```python
from build123d import *

# Parameters (mm, degrees)
ESQUISSE1_W        = 45
ESQUISSE1_H        = 60
BOSS_EXTRU_1_DEPTH = 5


with BuildPart() as part:
    # Esquisse1 → Boss.-Extru.1 (new body)
    with BuildSketch(Plane.XY):
        Polygon((112.625631329, 137.374368671), (100, 150), (-100, 150), (-112.625631329, 137.374368671), (-98.483495706, 123.232233047), (-123.232233047, 98.483495706), (-137.374368671, 112.625631329), (-150, 100), (-150, -100), (-137.374368671, -112.625631329), (-123.232233047, -98.483495706), (-98.483495706, -123.232233047), (-112.625631329, -137.374368671), (-100, -150), (100, -150), (112.625631329, -137.374368671), (98.483495706, -123.232233047), (123.232233047, -98.483495706), (137.374368671, -112.625631329), (150, -100), (150, 100), (137.374368671, 112.625631329), (123.232233047, 98.483495706), (98.483495706, 123.232233047), align=None)
        Rectangle(ESQUISSE1_W, ESQUISSE1_H, mode=Mode.SUBTRACT)
    extrude(amount=BOSS_EXTRU_1_DEPTH)


solid = part.part
```
Work out the finished part from the listing and answer in its coordinate system (mm). A direction names the side the tool comes from. Round coordinates to 2 decimals unless told otherwise and drop trailing zeros. Order: outer loops, then holes, each group sorted by start corner. A loop starts at its lowest first (then second) coordinate and runs counter-clockwise, first axis right, second up.
Q1. A cutting plane is placed at C-C, the plane z = 2.5. Determine the outline of the cut face in (x, y).
Solution:
outline: (-150, -100) - (-137.37, -112.63) - (-123.23, -98.48) - (-98.48, -123.23) - (-112.63, -137.37) - (-100, -150) - (100, -150) - (112.63, -137.37) - (98.48, -123.23) - (123.23, -98.48) - (137.37, -112.63) - (150, -100) - (150, 100) - (137.37, 112.63) - (123.23, 98.48) - (98.48, 123.23) - (112.63, 137.37) - (100, 150) - (-100, 150) - (-112.63, 137.37) - (-98.48, 123.23) - (-123.23, 98.48) - (-137.37, 112.63) - (-150, 100) - close; hole (-22.5, -30) - (22.5, -30) - (22.5, 30) - (-22.5, 30) - close
Q2. The mould has two halves that part along X. Classify faces 1 (the flat face through (144, 106, 2)), 2 (the flat face through (-144, 106, 2)), 3 (the flat face through (130.4, 105.65, 2.46)): pulls with the +X half, pulls with the -X half, needs draft (parallel to the pull), parting line crosses it, or undercut.
Solution:
face 1: pulls with the +X half
face 2: pulls with the -X half
face 3: undercut
Q3. A cutting plane is placed at A-A, the plane x = -8. Determine the outline of the cut face in (y, z), then the cut area to 3 significant figures.
Solution:
outline: (-150, 0) - (-30, 0) - (-30, 5) - (-150, 5) - close; (30, 0) - (150, 0) - (150, 5) - (30, 5) - close
area: 1,200 mm2
Q4. A cutting plane is placed at B-B, the plane y = 7. Determine the outline of the cut face in (x, z).
Solution:
outline: (-150, 0) - (-22.5, 0) - (-22.5, 5) - (-150, 5) - close; (22.5, 0) - (150, 0) - (150, 5) - (22.5, 5) - close
Q5. A tool of negligible diameter and unlimited length cuts with its end or side. For faces 4 (the flat face through (-105.456, -130.204, 2.465)), 5 (the flat face through (-144, -106, 2)), 6 (the flat face through (-130.4, -105.65, 2.46)), 7 (the flat face through (110.685, -111.031, 2.465)), 8 (the flat face through (105.65, -130.4, 2.46)), from which of +Z, -Z, +X, -X, +Y, -Y can it reach the whole face along a straight path? Write none if from no direction.
Solution:
face 4: +Z, -Z, -X
face 5: +Z, -Z, -X, -Y
face 6: +Z, -Z, -Y
face 7: +Z, -Z
face 8: +Z, -Z, +X
Q6. Find the intervals of material crossed by line 1 along X through (y, z) = (-5, 3.1); line 2 along Y through (x, z) = (-105, 3.3); line 3 along Y through (x, z) = (4, 1.65), in increasing order.
Solution:
line 1: x = -150 to -22.5, 22.5 to 150
line 2: y = -145 to -129.75, -116.72 to 116.72, 129.75 to 145
line 3: y = -150 to -30, 30 to 150
